Geometry: see drawing. Coordinates: mm, zero at the bounding-box minimum. Give positions to 0.01 mm unless a question says otherwise; leave off trailing zeros. Write each loop counter-clockwise with the first axis right and the second up, starting at its lowest first coordinate (ties: lowest second). Pieces come first, ordered by that corner, then holes.
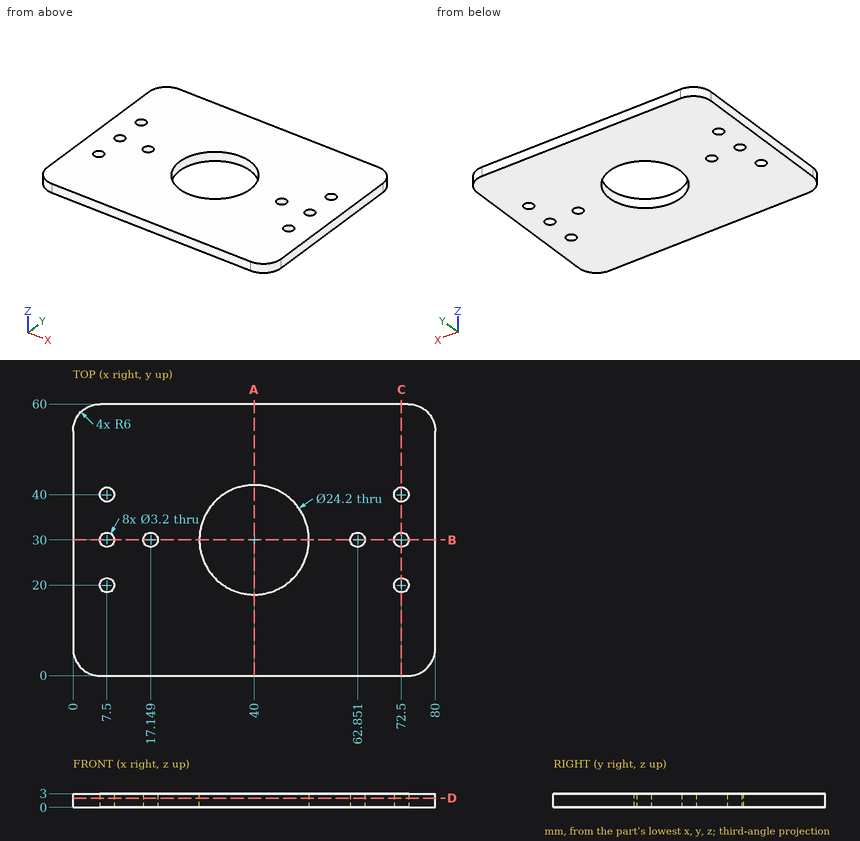
1. Section query D-D (z = 2). Give the number of separate pieces and of enclosed holes in the cut face, plus the area to 3 significant figures.
2. Section query C-C (x = 72.5). Return loops of the section in (y, z).
3. Section query B-B (y = 30). Return loops of the section in (x, z), plus the area to 3 significant figures.
4. Line query: probe 1 along Y at (x, z) = (7.5, 1.55); probe 2 along X at (y, z) = (19.5, 0.8); probe 3 along Y at (x, z) = (40, 2.3). Output: solid intervals per line, ascending.
5. Section query A-A (x = 40). Return loops of the section in (y, z), plus the area to 3 significant figures.
The answers:
1. separate pieces: 1
1. enclosed holes: 9
1. area: 4,240 mm2
2. outline: (0, 0) - (18.4, 0) - (18.4, 3) - (0, 3) - close; (21.6, 0) - (28.4, 0) - (28.4, 3) - (21.6, 3) - close; (31.6, 0) - (38.4, 0) - (38.4, 3) - (31.6, 3) - close; (41.6, 0) - (60, 0) - (60, 3) - (41.6, 3) - close
3. outline: (0, 0) - (5.9, 0) - (5.9, 3) - (0, 3) - close; (9.1, 0) - (15.55, 0) - (15.55, 3) - (9.1, 3) - close; (18.75, 0) - (27.9, 0) - (27.9, 3) - (18.75, 3) - close; (52.1, 0) - (61.25, 0) - (61.25, 3) - (52.1, 3) - close; (64.45, 0) - (70.9, 0) - (70.9, 3) - (64.45, 3) - close; (74.1, 0) - (80, 0) - (80, 3) - (74.1, 3) - close
3. area: 129 mm2
4. probe 1: y = 0 to 18.4, 21.6 to 28.4, 31.6 to 38.4, 41.6 to 60
4. probe 2: x = 0 to 5.98, 9.02 to 33.99, 46.01 to 70.98, 74.02 to 80
4. probe 3: y = 0 to 17.9, 42.1 to 60
5. outline: (0, 0) - (17.9, 0) - (17.9, 3) - (0, 3) - close; (42.1, 0) - (60, 0) - (60, 3) - (42.1, 3) - close
5. area: 107 mm2
